from build123d import *

# Parameters (mm, degrees)
F1_DEPTH = 10
F2_DEPTH = 10
F3_DEPTH = 30


with BuildPart() as f1:
    # F0 (on Front) → F1 (new body)
    with BuildSketch(Plane.XZ):
        with BuildLine():
            Line((-12.7058480853, 41.598128256), (-10.2291550788, 41.2866124053))
            ThreePointArc((-10.2291550788, 41.2866124053), (-9.1067668118, 42.6821747975), (-8.7058480853, 44.4276300352))
            ThreePointArc((-8.7058480853, 44.4276300352), (-8.8812998063, 45.5993085158), (-9.3922633163, 46.6682004935))
            Line((-9.3922633163, 46.6682004935), (-12.7058480853, 47.084979713))
            Line((-12.7058480853, 47.084979713), (-12.7058480853, 41.598128256))
        make_face()
        with BuildLine():
            ThreePointArc((-11.7422820262, 48.3098382277), (-16.6161256775, 43.5851757919), (-10.2291550788, 41.2866124053))
            Line((-10.2291550788, 41.2866124053), (-12.7058480853, 41.598128256))
            Line((-12.7058480853, 41.598128256), (-12.7058480853, 47.084979713))
            Line((-12.7058480853, 47.084979713), (-11.7422820262, 48.3098382277))
        make_face()
        with BuildLine():
            ThreePointArc((-9.3922633163, 46.6682004935), (-10.4151607617, 47.7067688834), (-11.7422820262, 48.3098382277))
            Line((-11.7422820262, 48.3098382277), (-12.7058480853, 47.084979713))
            Line((-12.7058480853, 47.084979713), (-9.3922633163, 46.6682004935))
        make_face()
    extrude(amount=F1_DEPTH)

    # F0 (on Front) → F2 (join)
    with BuildSketch(Plane.XZ):
        with BuildLine():
            Line((-10.2291550788, 41.2866124053), (0, 40))
            Line((0, 40), (16.6241960095, 30.8002115765))
            Line((16.6241960095, 30.8002115765), (19.0451929631, 35.175))
            Line((19.0451929631, 35.175), (0, 45.486851457))
            Line((0, 45.486851457), (-6.9169276979, 46.3568553736))
            Line((-6.9169276979, 46.3568553736), (-9.3922633163, 46.6682004935))
            ThreePointArc((-9.3922633163, 46.6682004935), (-8.8812998063, 45.5993085158), (-8.7058480853, 44.4276300352))
            ThreePointArc((-8.7058480853, 44.4276300352), (-9.1067668118, 42.6821747975), (-10.2291550788, 41.2866124053))
        make_face()
        with BuildLine():
            Line((12.0256917617, 78.5230289018), (-11.7422820262, 48.3098382277))
            ThreePointArc((-11.7422820262, 48.3098382277), (-10.4151607617, 47.7067688834), (-9.3922633163, 46.6682004935))
            Line((-9.3922633163, 46.6682004935), (-6.9169276979, 46.3568553736))
            Line((-6.9169276979, 46.3568553736), (15.9554479103, 75.4315864209))
            Line((15.9554479103, 75.4315864209), (12.0256917617, 78.5230289018))
        make_face()
    extrude(amount=F2_DEPTH)

    # F0 (on Front) → F3 (join)
    with BuildSketch(Plane.XZ):
        with BuildLine():
            Line((-12.7058480853, 41.598128256), (-10.2291550788, 41.2866124053))
            ThreePointArc((-10.2291550788, 41.2866124053), (-9.1067668118, 42.6821747975), (-8.7058480853, 44.4276300352))
            ThreePointArc((-8.7058480853, 44.4276300352), (-8.8812998063, 45.5993085158), (-9.3922633163, 46.6682004935))
            Line((-9.3922633163, 46.6682004935), (-12.7058480853, 47.084979713))
            Line((-12.7058480853, 47.084979713), (-12.7058480853, 41.598128256))
        make_face()
        with BuildLine():
            ThreePointArc((-9.3922633163, 46.6682004935), (-10.4151607617, 47.7067688834), (-11.7422820262, 48.3098382277))
            Line((-11.7422820262, 48.3098382277), (-12.7058480853, 47.084979713))
            Line((-12.7058480853, 47.084979713), (-9.3922633163, 46.6682004935))
        make_face()
        with BuildLine():
            ThreePointArc((-11.7422820262, 48.3098382277), (-16.6161256775, 43.5851757919), (-10.2291550788, 41.2866124053))
            Line((-10.2291550788, 41.2866124053), (-12.7058480853, 41.598128256))
            Line((-12.7058480853, 41.598128256), (-12.7058480853, 47.084979713))
            Line((-12.7058480853, 47.084979713), (-11.7422820262, 48.3098382277))
        make_face()
    extrude(amount=-F3_DEPTH)


solid = f1.part
Verification items for the finished model (mm, model axes). A direction names the side the tool comes from. Coordinates: 2 decimals unless noted, no trailing zeros. Write each loop counter-clockwise with the first axis right and the second up, starting at its lowest first coordinate (ties: lowest second). Pieces come first, ordered by that corner, then holes. Notation, with made-up numbers: M 74.5,-36 L 103.5,-36 A25 ccw 103.5,-17 Z; hole C 54,-24.75 d10. An arc over 180 degrees is marked long. Use CSV: the item, a comma, the result in double quotes.
Q1. Section check A-A, the plane x = 14. Enter the section's corners in (y, z), and give its area (3 significant figures).
Computed values:
outline,"M -10,32.25 L 0,32.25 L 0,37.91 L -10,37.91 Z; M -10,72.95 L 0,72.95 L 0,76.97 L -10,76.97 Z"
area,"96.8 mm²"
Q2. Set-up check for faces 5 (the flat face through (4.36, -4.93, 60.69)), 6 (the flat face through (1, -10, 57)): record each of +Z, -Z, +X, -X, +Y, -Y from which the full face is reachable in a straight line by a thin tool's end or side.
Computed values:
face 5,"+X, +Y, -Y"
face 6,"+Z, -Z, +X, -X, -Y"
Q3. Section check B-B, the plane y = -2. Enter the section's corners in (x, z) (3 decimals), and give its area (3 significant figures).
Computed values:
outline,"M -11.742,48.31 A4 ccw long -10.229,41.287 L 0,40 L 16.624,30.8 L 19.045,35.175 L 0,45.487 L -6.917,46.357 L 15.955,75.432 L 12.026,78.523 Z"
area,"390 mm²"
Q4. Go/stop test with flat-tipped pins: P1, Ø15.5, axis at x = -3, z = 62.5, coming from the +Y side; P2, Ø1, axis at y = 26, z = 44, coming from the +X side; P3, Ø2, axis at x = 1, z = 53.5, coming from the +Y side; P4, Ø6, axis at y = 14.5, z = 50, coming from the +X side. Record where each tip stops, or that it passes through.
Computed values:
P1,"y = 0"
P2,"x = -8.71"
P3,"through"
P4,"x = -9.64"
Q5. Section check C-C, the plane z = 43. Enter the section's corners in (x, y).
Computed values:
outline,"M -16.44,-10 L 4.59,-10 L 4.59,0 L -8.97,0 L -8.97,30 L -16.44,30 Z"
Q6. Mould release check, pull along X, two halves, no side actions. Record for faces 1 (the flat face through (-13, 30, 44)), 2 (the flat face through (-3.41, -4.93, 45.916)), 3 (the flat face through (-5.186, -4.93, 40.652)), 4 (the flat face through (8.2, -4.93, 35.46)): pulls with the +X half, pulls with the -X half, needs draft (parallel to the pull), parting line crosses it, or undercut.
Computed values:
face 1,"needs draft"
face 2,"pulls with the +X half"
face 3,"undercut"
face 4,"pulls with the -X half"
Q7. Section check D-D, the plane x = 6.5. Enter the section's corners in (y, z), and give its area (3 significant figures).
Computed values:
outline,"M -10,36.4 L 0,36.4 L 0,41.97 L -10,41.97 Z; M -10,63.41 L 0,63.41 L 0,71.5 L -10,71.5 Z"
area,"137 mm²"
Q8. Thickness scan on line 1 along Y through (x, z) = (7, 68.5); line 2 along Z through (x, y) = (9.5, -2); line 3 along Z through (x, y) = (15, -1). Record the ranges inside material, lowest first. Write a range as [from, to].
Computed values:
line 1,"[-10, 0]"
line 2,"[34.74, 40.34], [67.23, 75.31]"
line 3,"[31.7, 37.37], [74.22, 76.18]"
